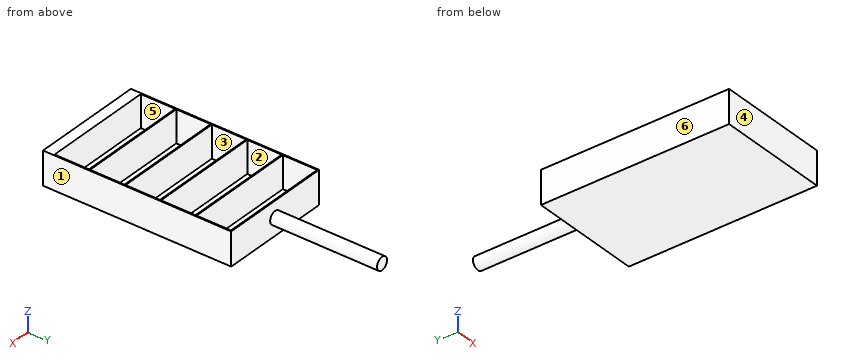
```python
from build123d import *

# Parameters (mm, degrees)
CROQUIS1_W              = 1050
CROQUIS1_H              = 1760
SALIENTE_EXTRUIR1_DEPTH = 10
CROQUIS2_W              = 1050
CROQUIS2_H              = 1760
CROQUIS2_W_2            = 1030
CROQUIS2_H_2            = 322
SALIENTE_EXTRUIR2_DEPTH = 300
CROQUIS3_R              = 59.221994718
SALIENTE_EXTRUIR3_DEPTH = 1000


with BuildPart() as part:
    # Croquis1 → Saliente-Extruir1 (new body)
    with BuildSketch(Plane.XY):
        Rectangle(CROQUIS1_W, CROQUIS1_H)
    extrude(amount=SALIENTE_EXTRUIR1_DEPTH)

    # Croquis2 → Saliente-Extruir2 (add)
    with BuildSketch(Plane.XY.offset(10)):
        Rectangle(CROQUIS2_W, CROQUIS2_H)
        with Locations((0, 377)):
            Rectangle(CROQUIS2_W_2, CROQUIS2_H_2, mode=Mode.SUBTRACT)
        with Locations((0, 709)):
            Rectangle(CROQUIS2_W_2, CROQUIS2_H_2, mode=Mode.SUBTRACT)
        with Locations((0, 45)):
            Rectangle(CROQUIS2_W_2, CROQUIS2_H_2, mode=Mode.SUBTRACT)
        with Locations((0, -287)):
            Rectangle(CROQUIS2_W_2, CROQUIS2_H_2, mode=Mode.SUBTRACT)
        with Locations((0, -619)):
            Rectangle(CROQUIS2_W_2, CROQUIS2_H_2, mode=Mode.SUBTRACT)
    extrude(amount=SALIENTE_EXTRUIR2_DEPTH)

    # Croquis3 → Saliente-Extruir3 (add)
    with BuildSketch(Plane(origin=(0, 880, 0), x_dir=(1, 0, 0), z_dir=(0, 1, 0))):
        with Locations(Location((0, -160.46266829, 0), (0, 0, 90))):
            Circle(CROQUIS3_R)
    extrude(amount=SALIENTE_EXTRUIR3_DEPTH)


solid = part.part
```
Design review of the part built by this model. Coordinates are the model's own, in mm. Face numbers are marked on the shaded views. A direction names the side the tool comes from. Give positions to 0.01 mm unless a question says otherwise; leave off trailing zeros. Order: outer loops, then holes, each group sorted by start corner. A loop starts at its lowest first (then second) coordinate and runs counter-clockwise, first axis right, second up. Notation, with made-up numbers: (20.25, 80.25) - (27.25, 80.25) arc R6 ccw to (27.25, 87.25) - close; hole circle Ø11 at (55.5, 44). An arc over 180 degrees is marked (long way). Use a Markdown table: item, result. Add a question column.
(1) Machinability: for the marked faces 5 and 6, which of the approach directions +Z, -Z, +X, -X, +Y, -Y give a long, thin tool a straight path to every point of the face, cutting with its end or side? Answer none if there is none.
(2) Add section A-A on x = 0. Give the boundary of the cut face in (y, z), then the cut area to 3 significant figures.
(3) Add section D-D on x = -111. Give the boundary of the cut face in (y, z).
(4) Add section B-B on z = 61. Give the boundary of the cut face in (x, y), then the cut area to 3 significant figures.
(5) Clearance check with flat-ended pins moving along their axes: P1, Ø5, axis at x = -72.5, z = 248.5, coming from the +Y side; P2, Ø5, axis at x = -216.5, y = 783, coming from the +Z side. State where each tip first meets the part, or that it passes through.
(6) Mouldability with a two-part tool opening along X and no side actions: class the marked faces 1, 2, 3 and 4 as +X half, -X half, draft (parallel to the pull), parting line (faces both ways), or undercut.
(7) Add section C-C on y = 761. Give the boundary of the cut face in (x, z), then the cut area to 3 significant figures.
(8) Wall thickness on probe 1 along Y at (x, z) = (-153, 81); probe 2 along X at (y, z) = (-519.5, 141); probe 3 along Y at (x, z) = (-8.5, 105): over which ranges is each line inside the solid? List them lowest first. Write a range as [from, to].
Report:
| question | item | result |
|---|---|---|
| 1 | face 5 | +Z |
| 1 | face 6 | +Z, -Z, -X, +Y, -Y |
| 2 | outline | (-880, 0) - (880, 0) - (880, 101.24) - (1880, 101.24) - (1880, 219.68) - (880, 219.68) - (880, 310) - (870, 310) - (870, 10) - (548, 10) - (548, 310) - (538, 310) - (538, 10) - (216, 10) - (216, 310) - (206, 310) - (206, 10) - (-116, 10) - (-116, 310) - (-126, 310) - (-126, 10) - (-448, 10) - (-448, 310) - (-458, 310) - (-458, 10) - (-780, 10) - (-780, 310) - (-880, 310) - close |
| 2 | area | 181,000 mm² |
| 3 | outline | (-880, 0) - (880, 0) - (880, 310) - (870, 310) - (870, 10) - (548, 10) - (548, 310) - (538, 310) - (538, 10) - (216, 10) - (216, 310) - (206, 310) - (206, 10) - (-116, 10) - (-116, 310) - (-126, 310) - (-126, 10) - (-448, 10) - (-448, 310) - (-458, 310) - (-458, 10) - (-780, 10) - (-780, 310) - (-880, 310) - close |
| 4 | outline | (-525, -880) - (525, -880) - (525, 880) - (-525, 880) - close; hole (-515, -780) - (515, -780) - (515, -458) - (-515, -458) - close; hole (-515, -448) - (515, -448) - (515, -126) - (-515, -126) - close; hole (-515, -116) - (515, -116) - (515, 206) - (-515, 206) - close; hole (-515, 216) - (515, 216) - (515, 538) - (-515, 538) - close; hole (-515, 548) - (515, 548) - (515, 870) - (-515, 870) - close |
| 4 | area | 190,000 mm² |
| 5 | P1 | stops at y = 880 |
| 5 | P2 | stops at z = 10 |
| 6 | face 1 | +X half |
| 6 | face 2 | undercut |
| 6 | face 3 | undercut |
| 6 | face 4 | draft |
| 7 | outline | (-525, 0) - (525, 0) - (525, 310) - (515, 310) - (515, 10) - (-515, 10) - (-515, 310) - (-525, 310) - close |
| 7 | area | 16,500 mm² |
| 8 | probe 1 | y = [-880, -780], [-458, -448], [-126, -116], [206, 216], [538, 548], [870, 880] |
| 8 | probe 2 | x = [-525, -515], [515, 525] |
| 8 | probe 3 | y = [-880, -780], [-458, -448], [-126, -116], [206, 216], [538, 548], [870, 1880] |
